Check sheet for the modelled part. Datum: model origin and axes. Units: mm. A direction names the side the tool comes from. Round coordinates to 2 decimals unless told otherwise and drop trailing zeros. Order: outer loops, then holes, each group sorted by start corner. A loop starts at its lowest first (then second) coordinate and runs counter-clockwise, first axis right, second up. Notation, with made-up numbers: (66, -9.5) -> (89, -9.5) arc R17 cw to (89, 21.5) -> close; hole circle Ø11 at (43.25, 48.5). An arc over 180 degrees is marked (long way). Answer in a Markdown table with one row per item.
from build123d import *

# Parameters (mm, degrees)
F0_R     = 3.175
F1_DEPTH = 12.7
F0_R_2   = 1.5875


with BuildPart() as f1:
    # F0 (on Front) → F1 (new body)
    with BuildSketch(Plane.XZ):
        with Locations((-96.8591794372, -59.9242933095)):
            Circle(F0_R)
    extrude(amount=F1_DEPTH)


with BuildPart() as f1b:
    # F0 (on Front) → F1, piece 2 (new body)
    with BuildSketch(Plane.XZ):
        with BuildLine():
            ThreePointArc((9.525, 0), (-0.4768479324, 9.5130563464), (-9.4772553384, -0.9525))
            ThreePointArc((-9.4772553384, -0.9525), (-6.2623833816, -7.1769199091), (0.3401785714, -9.5189234444))
            ThreePointArc((0.3401785714, -9.5189234444), (6.8544082857, -6.6138273378), (9.525, 0))
        make_face()
        Circle(F0_R, mode=Mode.SUBTRACT)
        with BuildLine():
            ThreePointArc((52.3875, 0), (50.1620069047, 5.5115227815), (44.7334821429, 7.9324362036))
            ThreePointArc((44.7334821429, 7.9324362036), (36.5125, 0), (44.7334821429, -7.9324362036))
            ThreePointArc((44.7334821429, -7.9324362036), (50.1620069047, -5.5115227815), (52.3875, 0))
        make_face()
        with Locations((44.45, 0)):
            Circle(F0_R, mode=Mode.SUBTRACT)
        with BuildLine():
            Line((11.3411865923, 17.5933818124), (15.7954255641, 61.9125))
            ThreePointArc((15.7954255641, 61.9125), (0, 47.625), (-15.7954255641, 61.9125))
            Line((-15.7954255641, 61.9125), (-9.4772553384, -0.9525))
            ThreePointArc((-9.4772553384, -0.9525), (-0.4768479324, 9.5130563464), (9.525, 0))
            ThreePointArc((9.525, 0), (6.8544082857, -6.6138273378), (0.3401785714, -9.5189234444))
            Line((0.3401785714, -9.5189234444), (44.7334821429, -7.9324362036))
            ThreePointArc((44.7334821429, -7.9324362036), (36.5125, 0), (44.7334821429, 7.9324362036))
            Line((44.7334821429, 7.9324362036), (18.9676000005, 8.8532337108))
            ThreePointArc((18.9676000005, 8.8532337108), (13.2611998974, 11.5713591498), (11.3411865923, 17.5933818124))
        make_face()
        with BuildLine():
            ThreePointArc((0, 79.375), (10.5003255158, 75.40625), (15.7504882737, 65.484375))
            Line((15.7504882737, 65.484375), (9.4502929642, 115.490625))
            ThreePointArc((9.4502929642, 115.490625), (9.5063048942, 114.896483242), (9.525, 114.3))
            ThreePointArc((9.525, 114.3), (6.7351920908, 107.5648079092), (0, 104.775))
            Line((0, 104.775), (0, 100.0252))
            Line((0, 100.0252), (0, 79.375))
        make_face()
        with BuildLine():
            ThreePointArc((9.525, 114.3), (9.5063048942, 114.896483242), (9.4502929642, 115.490625))
            ThreePointArc((9.4502929642, 115.490625), (0, 123.825), (-9.4502929642, 115.490625))
            ThreePointArc((-9.4502929642, 115.490625), (-7.14375, 107.9998046905), (0, 104.775))
            ThreePointArc((0, 104.775), (6.7351920908, 107.5648079092), (9.525, 114.3))
        make_face()
        with BuildLine():
            ThreePointArc((3.175, 114.3), (2.2450640303, 112.0549359697), (0, 111.125))
            ThreePointArc((0, 111.125), (-2.2450640303, 116.5450640303), (3.175, 114.3))
        make_face(mode=Mode.SUBTRACT)
        with BuildLine():
            ThreePointArc((15.7954255641, 61.9125), (15.8550939106, 62.7052534459), (15.875, 63.5))
            ThreePointArc((15.875, 63.5), (15.8438414904, 64.4941387366), (15.7504882737, 65.484375))
            ThreePointArc((15.7504882737, 65.484375), (10.5003255158, 75.40625), (0, 79.375))
            ThreePointArc((0, 79.375), (-10.5003255158, 75.40625), (-15.7504882737, 65.484375))
            ThreePointArc((-15.7504882737, 65.484375), (-15.8737438155, 63.6997054867), (-15.7954255641, 61.9125))
            ThreePointArc((-15.7954255641, 61.9125), (0, 47.625), (15.7954255641, 61.9125))
        make_face()
        with BuildLine():
            ThreePointArc((3.175, 63.5), (-2.2450640303, 61.2549359697), (0, 66.675))
            ThreePointArc((0, 66.675), (2.2450640303, 65.7450640303), (3.175, 63.5))
        make_face(mode=Mode.SUBTRACT)
        with BuildLine():
            ThreePointArc((-15.7504882737, 65.484375), (-10.5003255158, 75.40625), (0, 79.375))
            Line((0, 79.375), (0, 100.0252))
            Line((0, 100.0252), (0, 104.775))
            ThreePointArc((0, 104.775), (-7.14375, 107.9998046905), (-9.4502929642, 115.490625))
            Line((-9.4502929642, 115.490625), (-15.7504882737, 65.484375))
        make_face()
        with Locations((-1.5875, 100.0252)):
            Circle(F0_R_2, mode=Mode.SUBTRACT)
    extrude(amount=F1_DEPTH)


solid = f1b.part
Item 1: Cross-section at A-A (y = -5). State how many separate pieces and enclosed holes the cut face has, and give its area (3 significant figures).
Result sheet:
| item | result |
|---|---|
| separate pieces | 1 |
| enclosed holes | 5 |
| area | 3,800 mm^2 |
Item 2: Cross-section at B-B (x = 21). Record the boundary of the cut face in (y, z), and give its area (3 significant figures).
Result sheet:
| item | result |
|---|---|
| outline | (-12.7, -8.78) -> (0, -8.78) -> (0, 8.78) -> (-12.7, 8.78) -> close |
| area | 223 mm^2 |
Item 3: Cross-section at C-C (z = 45.5). Record the boundary of the cut face in (x, y), and give its area (3 significant figures).
Result sheet:
| item | result |
|---|---|
| outline | (-14.15, -12.7) -> (14.15, -12.7) -> (14.15, 0) -> (-14.15, 0) -> close |
| area | 359 mm^2 |
Item 4: Mould release check, pull along Z, two halves, no side actions. Record for faces 3 (the cylindrical face through (-15.873, -6.261, 63.725)), 4 (the flat face through (3, 0, 43)), 5 (the cylindrical face through (41.28, -6.26, 0.14)), 6 (the flat face through (13.537, -6.261, 39.443)): pulls with the +Z half, pulls with the -Z half, needs draft (parallel to the pull), parting line crosses it, or undercut.
Result sheet:
| item | result |
|---|---|
| face 3 | parting line crosses it |
| face 4 | needs draft |
| face 5 | undercut |
| face 6 | undercut |
Item 5: Depth check by flat-ended pin: P1, Ø1, axis at x = -6.5, z = 47, coming from the +Y side; P2, Ø5, axis at x = 0, z = 63.5, coming from the +Y side; P3, Ø3, axis at y = -10.5, z = 16.5, coming from the -X side; P4, Ø4, axis at x = 30, y = -10.5, coming from the -Z side. Enter the tip coordinate at first touch or a pass-through.
Result sheet:
| item | result |
|---|---|
| P1 | stops at y = 0 |
| P2 | passes through |
| P3 | stops at x = -11.38 |
| P4 | stops at z = -8.53 |
Item 6: Set-up check for faces 1 (the flat face through (-12.68, -6.26, 30.92)), 2 (the cylindrical face through (13.321, -6.261, 11.503)): record each of +Z, -Z, +X, -X, +Y, -Y from which the full face is reachable in a straight line by a thin tool's end or side.
Result sheet:
| item | result |
|---|---|
| face 1 | -Z, -X, +Y, -Y |
| face 2 | +X, +Y, -Y |
Item 7: Scan lines: line 1 (Z direction, x = 44.45, y = -4.75) (3 decimals); line 2 (Z direction, x = 1, y = -9); line 3 (Z direction, x = 2.5, y = -3.25). Record each from-to range of solid material in increasing order. Write a range as [from, to].
Result sheet:
| item | result |
|---|---|
| line 1 | z = [-7.943, -3.175], [3.175, 7.943] |
| line 2 | z = [-9.5, -3.01], [3.01, 60.49], [66.51, 111.29], [117.31, 123.77] |
| line 3 | z = [-9.44, -1.96], [1.96, 61.54], [65.46, 112.34], [116.26, 123.49] |
